Geometry check sheet. Reference: the model listing, model coordinates, mm. A direction names the side the tool comes from. Coordinates: 2 decimals unless noted, no trailing zeros. Write each loop counter-clockwise with the first axis right and the second up, starting at its lowest first coordinate (ties: lowest second). Pieces come first, ordered by that corner, then holes. Notation, with made-up numbers: (-19, 51.5) -> (10, 51.5) arc R29 cw to (10, 80.5) -> close; hole circle Ø7 at (19, 59). An arc over 180 degrees is marked (long way). Use a Markdown table: item, result.
```python
from build123d import *

# Parameters (mm, degrees)
SKETCH1_W      = 45.5
SKETCH1_H      = 37
BASIS_DEPTH    = 4
SKETCH3_R      = 8
HR04_GAT_DEPTH = 4


with BuildPart() as part:
    # Sketch1 → Basis (new body)
    with BuildSketch(Plane.XY):
        with Locations((22.75, 18.5)):
            Rectangle(SKETCH1_W, SKETCH1_H)
        Polygon((14.5, 39.5), (12.5, 37), (16.5, 37), align=None)
        Polygon((31, 39.5), (29, 37), (33, 37), align=None)
        Polygon((16.5, 0), (12.5, 0), (14.5, -2.5), align=None)
        Polygon((33, 0), (29, 0), (31, -2.5), align=None)
    extrude(amount=BASIS_DEPTH)

    # Sketch3 → HR04 gat (cut)
    with BuildSketch(Plane.XY.offset(4)):
        with Locations((9.8, 25.6)):
            Circle(SKETCH3_R)
        with Locations((35.7, 25.6)):
            Circle(SKETCH3_R)
    extrude(amount=-HR04_GAT_DEPTH, mode=Mode.SUBTRACT)


solid = part.part
```
Item 1: Thickness scan on L1, parallel to X at y = 26, z = 2; L2, parallel to Y at x = 9.8, z = 2.2; L3, parallel to X at y = 28, z = 3.5. Record the ranges inside material, lowest first. Write a range as [from, to].
Answer block:
| item | result |
|---|---|
| L1 | x = [0, 1.81], [17.79, 27.71], [43.69, 45.5] |
| L2 | y = [0, 17.6], [33.6, 37] |
| L3 | x = [0, 2.17], [17.43, 28.07], [43.33, 45.5] |
Item 2: Section check C-C on z = 1.85. Record the boundary of the cut face in (x, y).
Answer block:
| item | result |
|---|---|
| outline | (0, 0) -> (12.5, 0) -> (14.5, -2.5) -> (16.5, 0) -> (29, 0) -> (31, -2.5) -> (33, 0) -> (45.5, 0) -> (45.5, 37) -> (33, 37) -> (31, 39.5) -> (29, 37) -> (16.5, 37) -> (14.5, 39.5) -> (12.5, 37) -> (0, 37) -> close; hole circle Ø16 at (9.8, 25.6); hole circle Ø16 at (35.7, 25.6) |
Item 3: Section check A-A on x = 9.8. Record the boundary of the cut face in (y, z).
Answer block:
| item | result |
|---|---|
| outline | (0, 0) -> (17.6, 0) -> (17.6, 4) -> (0, 4) -> close; (33.6, 0) -> (37, 0) -> (37, 4) -> (33.6, 4) -> close |
Item 4: Mould release check, pull along Y, two halves, no side actions. Record for faces 6 (the cylindrical face through (40.001, 32.346, 2.028)), 7 (the flat face through (22, 14, 0)), 8 (the flat face through (30.014, 38.268, 1.972)): +Y half, -Y half, draft (parallel to the pull), parting line (faces both ways), or undercut.
Answer block:
| item | result |
|---|---|
| face 6 | undercut |
| face 7 | draft |
| face 8 | +Y half |
Item 5: Section check D-D on y = 25.6. Record the boundary of the cut face in (x, z), then the cut area to 3 significant figures.
Answer block:
| item | result |
|---|---|
| outline | (0, 0) -> (1.8, 0) -> (1.8, 4) -> (0, 4) -> close; (17.8, 0) -> (27.7, 0) -> (27.7, 4) -> (17.8, 4) -> close; (43.7, 0) -> (45.5, 0) -> (45.5, 4) -> (43.7, 4) -> close |
| area | 54.0 mm^2 |
Item 6: Depth check by flat-ended pin: P1, Ø1.2, axis at x = 25, z = 3, coming from the -Y side; P2, Ø9.5, axis at x = 35.7, y = 25.6, coming from the -Z side; P3, Ø1, axis at y = 32, z = 1.5, coming from the -X side; P4, Ø2, axis at x = 7, z = 2.5, coming from the +Y side. Enter the tip coordinate at first touch or a pass-through.
Answer block:
| item | result |
|---|---|
| P1 | stops at y = 0 |
| P2 | passes through |
| P3 | stops at x = 0 |
| P4 | stops at y = 37 |
Item 7: Tool access check on faces 1 (the flat face through (23, 0, 2)), 2 (the flat face through (6, 37, 2)), 3 (the flat face through (6, 0, 2)), 4 (the flat face through (39, 37, 2)), 5 (the flat face through (23, 37, 2)). Record the directions out of +Z, -Z, +X, -X, +Y, -Y that give a thin tool (end or side, any length) a straight path to the whole face; none if there is none.
Answer block:
| item | result |
|---|---|
| face 1 | +Z, -Z, -Y |
| face 2 | +Z, -Z, -X, +Y |
| face 3 | +Z, -Z, -X, -Y |
| face 4 | +Z, -Z, +X, +Y |
| face 5 | +Z, -Z, +Y |
Item 8: Section check B-B on y = 32. Record the boundary of the cut face in (x, z), then the cut area to 3 significant figures.
Answer block:
| item | result |
|---|---|
| outline | (0, 0) -> (5, 0) -> (5, 4) -> (0, 4) -> close; (14.6, 0) -> (30.9, 0) -> (30.9, 4) -> (14.6, 4) -> close; (40.5, 0) -> (45.5, 0) -> (45.5, 4) -> (40.5, 4) -> close |
| area | 105 mm^2 |
